```python
from build123d import *

# Parameters (mm, degrees)
SKETCH1_W           = 10.16
SKETCH1_H           = 10.16
BOSS_EXTRUDE1_DEPTH = 25.4
SKETCH2_W           = 7.62
SKETCH2_H           = 7.62
CUT_EXTRUDE1_DEPTH  = 26.4
SKETCH3_R           = 1.5
CUT_EXTRUDE2_DEPTH  = 3.54
SKETCH4_R           = 1.5
CUT_EXTRUDE3_DEPTH  = 3.54


with BuildPart() as part:
    # Sketch1 → Boss-Extrude1 (new body)
    with BuildSketch(Plane(origin=(0, 0, 0), x_dir=(0, 0, -1), z_dir=(1, 0, 0))):
        with Locations((5.08, 5.08)):
            Rectangle(SKETCH1_W, SKETCH1_H)
    extrude(amount=BOSS_EXTRUDE1_DEPTH)

    # Sketch2 → Cut-Extrude1 (cut, through all)
    with BuildSketch(Plane(origin=(25.4, 0, 0), x_dir=(0, 0, -1), z_dir=(1, 0, 0))):
        with Locations((3.81, 6.35)):
            Rectangle(SKETCH2_W, SKETCH2_H)
    extrude(amount=-CUT_EXTRUDE1_DEPTH, mode=Mode.SUBTRACT)

    # Sketch3 → Cut-Extrude2 (cut, through all)
    with BuildSketch(Plane.XY.offset(-7.62)):
        with Locations((7.62, 6.35)):
            Circle(SKETCH3_R)
        with Locations((17.78, 6.35)):
            Circle(SKETCH3_R)
    extrude(amount=-CUT_EXTRUDE2_DEPTH, mode=Mode.SUBTRACT)

    # Sketch4 → Cut-Extrude3 (cut, through all)
    with BuildSketch(Plane(origin=(0, 2.54, 0), x_dir=(1, 0, 0), z_dir=(0, 1, 0))):
        with Locations((2.54, 3.81)):
            Circle(SKETCH4_R)
        with Locations((22.86, 3.81)):
            Circle(SKETCH4_R)
        with Locations((12.7, 3.81)):
            Circle(SKETCH4_R)
    extrude(amount=-CUT_EXTRUDE3_DEPTH, mode=Mode.SUBTRACT)


solid = part.part
```
Can you work these out from the model? Positions are in its coordinate system, mm. A direction names the side the tool comes from. Give positions to 0.01 mm unless a question says otherwise; leave off trailing zeros. Loops run counter-clockwise (first coordinate to the right, second up) from the corner with the lowest first, then second, coordinate; pieces in that order, holes last. Notation, with made-up numbers: M 43.25,46 L 63.25,46 A24 cw 63.25,81 Z; hole C 0.25,48.25 d5. An arc over 180 degrees is marked long. Use CSV: the item, a comma, the result in double quotes. Start each with the question number.
1. Imagine slicing it at A-A, the plane x = 17.78. Write out the boundary of the cut face in (y, z), plus the area to 3 significant figures.
2. If I drill on L1, parallel to X at y = 1.95, z = -3.81; L2, parallel to Z at x = 2.54, y = 1.6; L3, parallel to Y at x = 7.62, z = -8.2, over which ranges is the centre line in solid material (lowest first)?
3. Imagine slicing it at C-C, the plane y = 5.75. Write out the boundary of the cut face in (x, z).
4. If we mould it in two halves opening along Y, with no side actions, what happens to faces 3 (the face through (6.12, 6.42, -8.87)), 4 (the face through (13, 0, -6)), 5 (the face through (13, 1, 0))? For each: released by +Y, released by -Y, zero draft, split by the parting line, or undercut.
5. Imagine slicing it at B-B, the plane z = -3.81. Write out the boundary of the cut face in (x, y), plus the area to 3 significant figures.
6. For P1, Ø2.5, axis at x = 7.62, y = 6.35, coming from the +Z side; P2, Ø4, axis at x = 10.5, y = 5, coming from the +Z side; P3, Ø2, axis at x = 5.5, z = -3.5, coming from the +Y side, each with a flat end and sliding along its axis, tell me the tip position at first contact or that it passes through.
7. Imagine slicing it at D-D, the plane z = -9.25. Write out the boundary of the cut face in (x, y), plus the area to 3 significant figures.
8. On a 3-axis mill with a long thin cutter (end or side, diameter ignored), from which of +Z, -Z, +X, -X, +Y, -Y can I reach the whole of each face in a straight line? I mean faces 1 (the face through (13, 5, -10.16)), 2 (the face through (13, 6, -7.62)). Say none if no direction works.
Response values:
1,outline,"M 0,-10.16 L 4.85,-10.16 L 4.85,-7.62 L 2.54,-7.62 L 2.54,0 L 0,0 Z; M 7.85,-10.16 L 10.16,-10.16 L 10.16,-7.62 L 7.85,-7.62 Z"
1,area,"37.5 mm^2"
2,L1,"0 to 1.04, 4.04 to 11.2, 14.2 to 21.36, 24.36 to 25.4"
2,L2,"-10.16 to -5.31, -2.31 to 0"
2,L3,"0 to 4.85, 7.85 to 10.16"
3,outline,"M 0,-10.16 L 6.25,-10.16 L 6.25,-7.62 L 0,-7.62 Z; M 8.99,-10.16 L 16.41,-10.16 L 16.41,-7.62 L 8.99,-7.62 Z; M 19.15,-10.16 L 25.4,-10.16 L 25.4,-7.62 L 19.15,-7.62 Z"
4,face 3,"undercut"
4,face 4,"released by -Y"
4,face 5,"zero draft"
5,outline,"M 0,0 L 1.04,0 L 1.04,2.54 L 0,2.54 Z; M 4.04,0 L 11.2,0 L 11.2,2.54 L 4.04,2.54 Z; M 14.2,0 L 21.36,0 L 21.36,2.54 L 14.2,2.54 Z; M 24.36,0 L 25.4,0 L 25.4,2.54 L 24.36,2.54 Z"
5,area,"41.7 mm^2"
6,P1,"through"
6,P2,"z = -7.62"
6,P3,"y = 2.54"
7,outline,"M 0,0 L 25.4,0 L 25.4,10.16 L 0,10.16 Z; hole C 7.62,6.35 d3; hole C 17.78,6.35 d3"
7,area,"244 mm^2"
8,face 1,"-Z, +X, -X, +Y, -Y"
8,face 2,"+Z, +X, -X, +Y"
